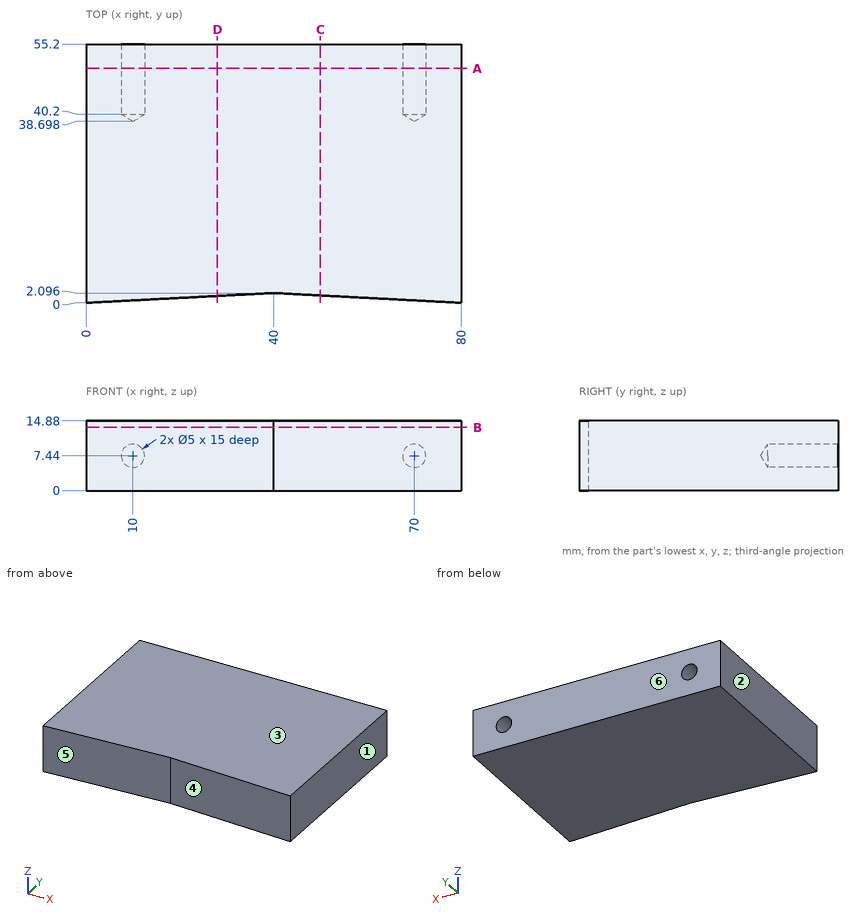
Job drawing, mm, ordinate dimensions from the low corner. One solid piece. A direction names the side the tool comes from. Coordinates: 2 decimals unless noted, no trailing zeros. Order: outer loops, then holes, each group sorted by start corner. A loop starts at its lowest first (then second) coordinate and runs counter-clockwise, first axis right, second up. Notation, with made-up numbers: (56, 60) - (107, 60) arc R23 ccw to (107, 81) - close; hole circle Ø4 at (53.25, -26). An arc over 180 degrees is marked (long way). Write each question's results on one line, items separated by ' | '. Start each with the question number.
Item 1: Band-saw the part on C-C on x = 50. Write the cut outline in (y, z).
Item 2: Band-saw the part on D-D on x = 28. Write the cut outline in (y, z).
Item 3: Flat gauge pin, fed straight in: pin 1 (4 mm diameter, centred on x = 70, z = 7.44, fed in from -Y). Where does the tip first touch, or does it go through?
Item 4: Band-saw the part on B-B on z = 13.5. Write the cut outline in (x, y).
Item 5: Band-saw the part on A-A on y = 50. Write the cut outline in (x, z), and give its area (3 significant figures).
Item 6: Wall check: probe 1 along Z at (x, y) = (70, 44); probe 2 along Y at (x, z) = (61, 12); probe 3 along Y at (x, z) = (16, 1.5). Give the ranges that are in metal, low to high. Write a range as [from, to].
Item 7: Mould opens along X. For the marked faces 1, 2, 3 and 4 say: released by +X, released by -X, zero draft, split by the parting line, or undercut.
Item 8: Tool access for the marked faces 5 and 6: list every direction of +Z, -Z, +X, -X, +Y, -Y with a clear straight run to the whole face (end or side of a thin tool).
Numbers:
1) outline: (1.57, 0) - (55.2, 0) - (55.2, 14.88) - (1.57, 14.88) - close
2) outline: (1.47, 0) - (55.2, 0) - (55.2, 14.88) - (1.47, 14.88) - close
3) pin 1: y = 0.42
4) outline: (0, 0) - (40, 2.1) - (80, 0) - (80, 55.2) - (0, 55.2) - close
5) outline: (0, 0) - (80, 0) - (80, 14.88) - (0, 14.88) - close; hole circle Ø5 at (10, 7.44); hole circle Ø5 at (70, 7.44) | area: 1,150 mm^2
6) probe 1: [0, 4.94], [9.94, 14.88] | probe 2: [1, 55.2] | probe 3: [0.84, 55.2]
7) face 1: released by +X | face 2: released by -X | face 3: zero draft | face 4: undercut
8) face 5: +Z, -Z, -Y | face 6: +Z, -Z, +X, -X, +Y
